Can you work these out from the model? Positions are in its coordinate system, mm. Coordinates: 2 decimals unless noted, no trailing zeros. Loops run counter-clockwise (first coordinate to the right, second up) from the corner with the lowest first, then second, coordinate; pieces in that order, holes last. Notation, with made-up numbers: M -13.75,-3 L 11.25,-3 A26 cw 11.25,20 Z; hole C -38.75,66.5 d7. An arc over 180 degrees is marked long. Answer as a JSON object with one key per item and string values. Group by question number.
Item 1: Suppose I cut it at B-B (x = 55). Write out the boundary of the cut face in (y, z), then the cut area to 3 significant figures.
Item 2: I'm going to push flat-ended pins straight in: pin 1 Ø3.5 at (x, z) = (106, 63) entering from +Y; pin 2 Ø2.5 at (x, z) = (21, 63) entering from -Y; pin 3 Ø2.5 at (x, z) = (27, 68.5) entering from -Y; pin 4 Ø4 at (x, y) = (105, 56) entering from +Z. Where does each tip first touch, or does it pass through?
Item 3: If I drill on line 1 (X direction, y = 116, z = 64); line 2 (Y direction, x = 20, z = 66.3); line 3 (Y direction, x = 105, z = 66), over which ranges is the centre line in solid material (lowest first)?
Item 4: Suppose I cut it at A-A (z = 63.25). Write out the boundary of the cut face in (x, y), then the cut area to 3 significant figures.
Item 5: Suppose I cut it at C-C (y = 116). Count the separate pieces of the cut face and the enclosed holes in it, then the cut area to 3 significant figures.
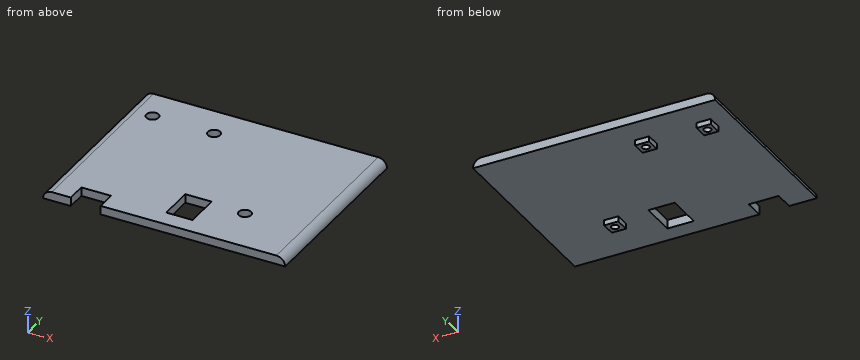
```python
from build123d import *

# Parameters (mm, degrees)
SKETCH1_W                = 150
SKETCH1_H                = 135
SKETCH1_R                = 2.1
BOSS_EXTRUDE2_DEPTH      = 70
SKETCH13_W               = 166.167800453
SKETCH13_H               = 148.934240363
CUT_EXTRUDE1_DEPTH       = 60
SKETCH17_W               = 17
SKETCH17_H               = 11
SKETCH17_W_2             = 15
SKETCH17_H_2             = 20
CUT_EXTRUDE5_DEPTH       = 10
CUT_EXTRUDE6_DEPTH       = 203.051973512
CUT_EXTRUDE6_DEPTH_BACK  = 203.051973512
SKETCH18_W               = 150
SKETCH18_H               = 135
CUT_EXTRUDE7_DEPTH       = 206.095744471
CUT_EXTRUDE7_DEPTH_BACK  = 206.095744471
FILLET1_R                = 5
SKETCH20_W               = 8
SKETCH20_H               = 8
BOSS_EXTRUDE3_DEPTH      = 3
CUT_EXTRUDE9_START       = -5
SKETCH21_R               = 3.5
SKETCH21_R_2             = 2.1
CUT_EXTRUDE9_DEPTH       = 5
CUT_EXTRUDE10_DEPTH      = 197.81971446
CUT_EXTRUDE10_DEPTH_BACK = 197.81971446
SKETCH21_2_R             = 2.1


with BuildPart() as part:
    # Sketch1 → Boss-Extrude2 (new body)
    with BuildSketch(Plane.XY):
        with Locations((75, 67.5)):
            Rectangle(SKETCH1_W, SKETCH1_H)
        with Locations((20, 116)):
            Circle(SKETCH1_R, mode=Mode.SUBTRACT)
        with Locations((55, 116)):
            Circle(SKETCH1_R, mode=Mode.SUBTRACT)
        with Locations((105, 56)):
            Circle(SKETCH1_R, mode=Mode.SUBTRACT)
    extrude(amount=BOSS_EXTRUDE2_DEPTH)

    # Sketch13 → Cut-Extrude1 (cut)
    with BuildSketch(Plane(origin=(0, 0, 0), x_dir=(-1, 0, 0), z_dir=(0, 0, -1))):
        with Locations((-76.451247165, 67.95351474)):
            Rectangle(SKETCH13_W, SKETCH13_H)
    extrude(amount=-CUT_EXTRUDE1_DEPTH, mode=Mode.SUBTRACT)

    # Sketch17 → Cut-Extrude5 (cut)
    with BuildSketch(Plane.XY.offset(70)):
        with Locations((29.68, 33.5)):
            Rectangle(SKETCH17_W, SKETCH17_H)
        with Locations((77.5, 48)):
            Rectangle(SKETCH17_W_2, SKETCH17_H_2)
    extrude(amount=-CUT_EXTRUDE5_DEPTH, mode=Mode.SUBTRACT)

    # Sketch18 → Cut-Extrude6 (cut, two sides: drawn at the far end of the back side and taken through both)
    # profile 1 of 2: a face of its own
    with BuildSketch(Plane.XY.offset(70).offset(-CUT_EXTRUDE6_DEPTH_BACK)):
        Polygon((-16.428571429, -29.414285714), (-20.085714286, 157.1), (193.857142857, 157.1), (193.857142857, -29.414285714), align=None)
        with Locations((75, 67.5)):
            Rectangle(SKETCH18_W, SKETCH18_H, mode=Mode.SUBTRACT)
    # profile 2 of 2: a face of its own
    with BuildSketch(Plane.XY.offset(70).offset(-CUT_EXTRUDE6_DEPTH_BACK)):
        Polygon((143, 28), (5.38, 28), (5.38, 135), (0, 135), (0, 0), (150, 0), (150, 135), (143, 135), align=None)
    extrude(amount=CUT_EXTRUDE6_DEPTH + CUT_EXTRUDE6_DEPTH_BACK, mode=Mode.SUBTRACT)

    # Sketch19 → Cut-Extrude7 (cut, two sides: drawn at the far end of the back side and taken through both)
    with BuildSketch(Plane(origin=(143, 0, 0), x_dir=(0, 0, -1), z_dir=(1, 0, 0)).offset(-CUT_EXTRUDE7_DEPTH_BACK)):
        Polygon((-65, 138.622751323), (-65, 12.247752415), (-38.78181863, -5.10096745), (-31.852947011, 142.632473856), align=None)
    extrude(amount=CUT_EXTRUDE7_DEPTH + CUT_EXTRUDE7_DEPTH_BACK, mode=Mode.SUBTRACT)

    # Fillet1
    fillet1_edges = [part.edges().sort_by_distance(p)[0] for p in [
        (5.38, 81.5, 70),
        (143, 81.5, 70),
    ]]
    fillet(fillet1_edges, radius=FILLET1_R - 0.0001)  # a hair under: the kernel refuses the full size

    # Sketch20 → Boss-Extrude3 (add)
    with BuildSketch(Plane(origin=(0, 0, 65), x_dir=(-1, 0, 0), z_dir=(0, 0, -1))):
        with Locations((-55, 116)):
            Rectangle(SKETCH20_W, SKETCH20_H)
        with Locations((-20, 116)):
            Rectangle(SKETCH20_W, SKETCH20_H)
        with Locations((-105, 56)):
            Rectangle(SKETCH20_W, SKETCH20_H)
    extrude(amount=BOSS_EXTRUDE3_DEPTH)

    # Sketch21 → Cut-Extrude9 (cut)
    # profile 1 of 3: a face of its own
    with BuildSketch(Plane.XY.offset(70).offset(CUT_EXTRUDE9_START)):
        with Locations((20, 116)):
            Circle(SKETCH21_R)
        with Locations((20, 116)):
            Circle(SKETCH21_R_2, mode=Mode.SUBTRACT)
    # profile 2 of 3: a face of its own
    with BuildSketch(Plane.XY.offset(70).offset(CUT_EXTRUDE9_START)):
        with Locations((55, 116)):
            Circle(SKETCH21_R)
        with Locations((55, 116)):
            Circle(SKETCH21_R_2, mode=Mode.SUBTRACT)
    # profile 3 of 3: a face of its own
    with BuildSketch(Plane.XY.offset(70).offset(CUT_EXTRUDE9_START)):
        with Locations((105, 56)):
            Circle(SKETCH21_R)
        with Locations((105, 56)):
            Circle(SKETCH21_R_2, mode=Mode.SUBTRACT)
    extrude(amount=CUT_EXTRUDE9_DEPTH, mode=Mode.SUBTRACT)

    # Sketch21<2> → Cut-Extrude10 (cut, two sides: drawn at the far end of the back side and taken through both)
    with BuildSketch(Plane.XY.offset(70).offset(-CUT_EXTRUDE10_DEPTH_BACK)):
        with Locations((20, 116)):
            Circle(SKETCH21_2_R)
        with Locations((55, 116)):
            Circle(SKETCH21_2_R)
        with Locations((105, 56)):
            Circle(SKETCH21_2_R)
    extrude(amount=CUT_EXTRUDE10_DEPTH + CUT_EXTRUDE10_DEPTH_BACK, mode=Mode.SUBTRACT)


solid = part.part
```
From the geometry:
{
 "1": {"outline": "M 28,65 L 112,65 L 112,62 L 113.9,62 L 113.9,65 L 112.5,65 L 112.5,70 L 28,70 Z; M 118.1,62 L 120,62 L 120,65 L 135,65 L 135,70 L 119.5,70 L 119.5,65 L 118.1,65 Z", "area": "511 mm2"},
 "2": {"pin 1": "y = 60", "pin 2": "y = 112", "pin 3": "y = 39", "pin 4": "through"},
 "3": {"line 1": "16 to 17.9, 22.1 to 24, 51 to 52.9, 57.1 to 59", "line 2": "28 to 112.5, 119.5 to 135", "line 3": "28 to 52.5, 59.5 to 135"},
 "4": {"outline": "M 16,112 L 24,112 L 24,120 L 16,120 Z; M 51,112 L 59,112 L 59,120 L 51,120 Z; M 101,52 L 109,52 L 109,60 L 101,60 Z; hole C 20,116 d4.2; hole C 55,116 d4.2; hole C 105,56 d4.2", "area": "150 mm2"},
 "5": {"separate pieces": "3", "enclosed holes": "0", "area": "630 mm2"}
}
